The model under review builds one solid part; all positions refer to its coordinate system, in mm. A direction names the side the tool comes from. Give positions to 0.01 mm unless a question says otherwise; leave off trailing zeros. Loops run counter-clockwise (first coordinate to the right, second up) from the corner with the lowest first, then second, coordinate; pieces in that order, holes last. Notation, with made-up numbers: M 6.25,83.25 L 23.25,83.25 A20 cw 23.25,114.25 Z; hole C -13,89 d9. An arc over 180 degrees is marked long. One line per item, written item: value. Start each with the question number.
Q1. Mouldability with a two-part tool opening along Z and no side actions: class faces 1 (the face through (9, 12, 8)), 2 (the face through (-9, 12, 8)), 3 (the face through (4, 0, 3.6)), 4 (the face through (0, -15, 3)) as released by +Z, released by -Z, zero draft, split by the parting line, or undercut.
Q2. To check wall thickness, follow line 1 along Y through (x, z) = (-6.75, 6); line 2 along Y through (x, z) = (0, 6.35); line 3 along Z through (x, y) = (-14, 4.25). State the ranges of each line that lie inside material, in increasing order. Write a range as from..to.
Q3. We need section D-D on z = 1.25. Write out the cut boundary in (x, y).
Q4. We need section B-B on x = 0. Write out the cut boundary in (y, z).
Q5. We need section C-C on x = 9. Write out the cut boundary in (y, z), plus the area to 4 significant figures.
Q6. For faces 5 (the face through (0, -6, 7)), 6 (the face through (-9.1, 9.5, 7.5)), 7 (the face through (15, 0, 4)), list the 3-axis set-ups (+Z, -Z, +X, -X, +Y, -Y) from which the entire face can be reached by the end or side of a thin tool; tool diameter is ignored.
Q7. We need section A-A on y = 0. Write out the cut boundary in (x, z).
Q8. For pin 1 (1.5 mm diameter, centred on x = 2.5, z = 8.5, fed in from -Y); pin 2 (11 mm diameter, centred on x = 5, y = -0.5, fed in from +Z), all flat-tipped, find the tip position at first contact; note any pin that passes through.
```python
from build123d import *

# Parameters (mm, degrees)
BASE_SKETCH_W           = 30
BASE_SKETCH_H           = 30
BASE_DEPTH              = 7
HIGHER_ADAPTER_SKETCH_W = 30
HIGHER_ADAPTER_SKETCH_H = 7.5
HIGHER_ADAPTER_DEPTH    = 3
MOUNT_SCREW_D           = 6.6
MOUNT_SCREW_CBORE_D     = 11
MOUNT_SCREW_CBORE_DEPTH = 3.4
BOTTOM_TIES_SKETCH_R    = 4
BOTTOM_TIES_SKETCH_R_2  = 2
BOTTOM_TIES_DEPTH       = 4
TOP_TIES_SKETCH_R       = 4
TOP_TIES_SKETCH_R_2     = 2
TOP_TIES_DEPTH          = 4
ROUNDING_R              = 3


with BuildPart() as part:
    # Base sketch → Base (new body)
    with BuildSketch(Plane.XY):
        Rectangle(BASE_SKETCH_W, BASE_SKETCH_H)
    extrude(amount=BASE_DEPTH)

    # Higher adapter sketch → Higher adapter (add)
    with BuildSketch(Plane.XY.offset(7)):
        with Locations((0, 11.25)):
            Rectangle(HIGHER_ADAPTER_SKETCH_W, HIGHER_ADAPTER_SKETCH_H)
    extrude(amount=HIGHER_ADAPTER_DEPTH)

    # Mount screw (through all)
    with Locations(Plane.XY.offset(7)):
        with Locations((0, 0)):
            CounterBoreHole(MOUNT_SCREW_D / 2, MOUNT_SCREW_CBORE_D / 2, MOUNT_SCREW_CBORE_DEPTH)

    # Bottom ties sketch → Bottom ties (cut)
    # profile 1 of 2: a face of its own
    with BuildSketch(Plane.XZ.offset(13.5)):
        with Locations((-9, 7)):
            Circle(BOTTOM_TIES_SKETCH_R)
        with Locations((-9, 7)):
            Circle(BOTTOM_TIES_SKETCH_R_2, mode=Mode.SUBTRACT)
    # profile 2 of 2: a face of its own
    with BuildSketch(Plane.XZ.offset(13.5)):
        with Locations((9, 7)):
            Circle(BOTTOM_TIES_SKETCH_R)
        with Locations((9, 7)):
            Circle(BOTTOM_TIES_SKETCH_R_2, mode=Mode.SUBTRACT)
    extrude(amount=-BOTTOM_TIES_DEPTH, mode=Mode.SUBTRACT)

    # Top ties sketch → Top ties (cut)
    # profile 1 of 2: a face of its own
    with BuildSketch(Plane(origin=(0, 13.5, 0), x_dir=(1, 0, 0), z_dir=(0, 1, 0))):
        with Locations((-9, -10)):
            Circle(TOP_TIES_SKETCH_R)
        with Locations((-9, -10)):
            Circle(TOP_TIES_SKETCH_R_2, mode=Mode.SUBTRACT)
    # profile 2 of 2: a face of its own
    with BuildSketch(Plane(origin=(0, 13.5, 0), x_dir=(1, 0, 0), z_dir=(0, 1, 0))):
        with Locations((9, -10)):
            Circle(TOP_TIES_SKETCH_R)
        with Locations((9, -10)):
            Circle(TOP_TIES_SKETCH_R_2, mode=Mode.SUBTRACT)
    extrude(amount=-TOP_TIES_DEPTH, mode=Mode.SUBTRACT)

    # Rounding
    rounding_edges = [part.edges().sort_by_distance(p)[0] for p in [
        (15, -15, 3.5),
        (-15, -15, 3.5),
        (-15, 15, 5),
        (15, 15, 5),
    ]]
    fillet(rounding_edges, radius=ROUNDING_R)


solid = part.part
```
Solved:
1. face 1: undercut
1. face 2: undercut
1. face 3: released by +Z
1. face 4: zero draft
2. line 1: -15..-13.5, -9.5..15
2. line 2: -15..-5.5, 5.5..15
2. line 3: 0..7
3. outline: M -15,-12 A3 ccw -12,-15 L 12,-15 A3 ccw 15,-12 L 15,12 A3 ccw 12,15 L -12,15 A3 ccw -15,12 Z; hole C 0,0 d6.6
4. outline: M -15,0 L -3.3,0 L -3.3,3.6 L -5.5,3.6 L -5.5,7 L -15,7 Z; M 3.3,0 L 15,0 L 15,10 L 7.5,10 L 7.5,7 L 5.5,7 L 5.5,3.6 L 3.3,3.6 Z
5. outline: M -15,0 L 15,0 L 15,10 L 7.5,10 L 7.5,7 L -15,7 Z; hole M -13.5,3 L -9.5,3 L -9.5,5 L -13.5,5 Z; hole M 9.5,6 L 13.5,6 L 13.5,8 L 9.5,8 Z
5. area: 216.5 mm2
6. face 5: +Z, +X, -X, -Y
6. face 6: none
6. face 7: +Z, -Z, +X, +Y, -Y
7. outline: M -15,0 L -3.3,0 L -3.3,3.6 L -5.5,3.6 L -5.5,7 L -15,7 Z; M 3.3,0 L 15,0 L 15,7 L 5.5,7 L 5.5,3.6 L 3.3,3.6 Z
8. pin 1: y = 7.5
8. pin 2: z = 7
